```python
from build123d import *

# Parameters (mm, degrees)
SKETCH1_W           = 7
SKETCH1_H           = 7
BOSS_EXTRUDE1_DEPTH = 3
CUT_EXTRUDE1_DEPTH  = 7
CUT_EXTRUDE2_DEPTH  = 11
SKETCH4_R           = 1.8
CUT_EXTRUDE3_DEPTH  = 0.8
CUT_EXTRUDE4_DEPTH  = 0.4


with BuildPart() as part:
    # Sketch1 → Boss-Extrude1 (new body)
    with BuildSketch(Plane(origin=(0, 0, 0), x_dir=(1, 0, 0), z_dir=(0, 1, 0))):
        with Locations((3.5, 3.5)):
            Rectangle(SKETCH1_W, SKETCH1_H)
    extrude(amount=BOSS_EXTRUDE1_DEPTH)

    # Sketch2 → Cut-Extrude1 (cut)
    with BuildSketch(Plane.XY):
        Polygon((0, 0), (0.7, 3), (0, 3), align=None)
        Polygon((7, 0), (6.3, 3), (7, 3), align=None)
    extrude(amount=-CUT_EXTRUDE1_DEPTH, mode=Mode.SUBTRACT)

    # Sketch3 → Cut-Extrude2 (cut)
    with BuildSketch(Plane(origin=(0, 0, 0), x_dir=(0, 0, -1), z_dir=(1, 0, 0))):
        Polygon((0, 0), (0.7, 3), (0, 3), align=None)
        Polygon((7, 3), (6.3, 3), (7, 0), align=None)
    extrude(amount=CUT_EXTRUDE2_DEPTH, mode=Mode.SUBTRACT)

    # Sketch4 → Cut-Extrude3 (cut)
    with BuildSketch(Plane.XZ):
        with Locations(Location((3.5, -3.5, 0), (0, 0, 270))):
            Circle(SKETCH4_R)
    extrude(amount=-CUT_EXTRUDE3_DEPTH, mode=Mode.SUBTRACT)

    # Sketch5 → Cut-Extrude4 (cut)
    with BuildSketch(Plane(origin=(0, 3, 0), x_dir=(1, 0, 0), z_dir=(0, 1, 0))):
        with BuildLine():
            Line((2.118256711, 5.29301719), (2.791333634, 5.29301719))
            Line((2.791333634, 5.29301719), (2.791333634, 3.393678247))
            add(Edge.make_bspline(
                [(2.791333634, 3.393678247), (2.79159059, 3.357687368), (2.792081143, 3.288977364), (2.792418818, 3.190811929), (2.794287554, 3.102674552), (2.798340091, 3.024423212), (2.801121459, 2.956097816), (2.806286157, 2.897685825), (2.811438338, 2.849209985), (2.816447496, 2.820376155), (2.818677384, 2.807540427)],
                knots=[0, 0, 0, 0, 1.470600056, 2.807515117, 4.011048972, 5.072079398, 6.00911328, 6.804506435, 7.467811572, 8, 8, 8, 8], degree=3))
            add(Edge.make_bspline(
                [(2.818677384, 2.807540427), (2.827870656, 2.772937179), (2.845973369, 2.704799015), (2.895871105, 2.611655954), (2.961785309, 2.529556211), (3.029020227, 2.471005878), (3.08983939, 2.429568298), (3.141500286, 2.404348789), (3.196312159, 2.381359585), (3.255433761, 2.363720163), (3.318230563, 2.348285034), (3.385461086, 2.339360335), (3.456557942, 2.33251085), (3.505290309, 2.331828921), (3.530316005, 2.331478728)],
                knots=[0, 0, 0, 0, 1.376921055, 2.711331395, 4.038631339, 5.418057255, 6.132954575, 6.870556231, 7.630397752, 8.422890386, 9.247036838, 10.121396817, 11.035274583, 12, 12, 12, 12], degree=3))
            add(Edge.make_bspline(
                [(3.530316005, 2.331478728), (3.555564197, 2.331936651), (3.604721911, 2.332828219), (3.67595983, 2.338137813), (3.742423591, 2.348155186), (3.804072535, 2.361289897), (3.86123227, 2.37788997), (3.913446785, 2.398907615), (3.960633797, 2.424200444), (4.016077825, 2.462322988), (4.075735526, 2.516101492), (4.133148446, 2.589220237), (4.174238425, 2.669935378), (4.193511366, 2.743634339), (4.203417011, 2.807845981), (4.209452062, 2.864033397), (4.214971422, 2.927618056), (4.219983422, 2.9984258), (4.223410988, 3.07650978), (4.225264898, 3.162067474), (4.226723935, 3.255085239), (4.227057995, 3.319592414), (4.22723107, 3.353013183)],
                knots=[0, 0, 0, 0, 1.036876239, 2.018776863, 2.930845756, 3.794842666, 4.605604932, 5.371924355, 6.101864688, 6.799283669, 8.1310906, 9.382718023, 10.597336334, 11.822035891, 12.492591141, 13.265194674, 14.141890321, 15.11351293, 16.179860579, 17.351049011, 18.627594861, 20, 20, 20, 20], degree=3))
            Line((4.22723107, 3.353013183), (4.22723107, 5.29301719))
            Line((4.22723107, 5.29301719), (4.900307993, 5.29301719))
            Line((4.900307993, 5.29301719), (4.900307993, 3.462388183))
            add(Edge.make_bspline(
                [(4.900307993, 3.462388183), (4.900221723, 3.411906909), (4.900055958, 3.314908527), (4.897467772, 3.175352057), (4.891967054, 3.047314846), (4.887360678, 2.930577419), (4.878475168, 2.825437586), (4.86917207, 2.731829975), (4.85718756, 2.649770945), (4.840097538, 2.556498932), (4.811376645, 2.451853735), (4.765088439, 2.336259695), (4.705930722, 2.231093862), (4.634139223, 2.135952726), (4.550127521, 2.050458146), (4.452637717, 1.97494623), (4.342672295, 1.908498965), (4.241901685, 1.860652783), (4.154042624, 1.828434731), (4.082482889, 1.806630998), (4.005897563, 1.788473049), (3.924376469, 1.774063102), (3.837884577, 1.761913385), (3.746390484, 1.753799365), (3.650032611, 1.748735644), (3.584309093, 1.748345307), (3.550648537, 1.748145395)],
                knots=[0, 0, 0, 0, 1.415574045, 2.719986624, 3.913607924, 5.00929969, 5.995467356, 6.871900228, 7.64671288, 8.320227872, 9.530145585, 10.682614022, 11.803571353, 12.90325401, 14.015460715, 15.154679255, 16.351678057, 17.612271512, 18.275764165, 18.974412946, 19.708786676, 20.481351116, 21.295095879, 22.157200529, 23.056203067, 24, 24, 24, 24], degree=3))
            add(Edge.make_bspline(
                [(3.550648537, 1.748145395), (3.510214347, 1.748662249), (3.431887293, 1.749663472), (3.318189063, 1.754129843), (3.212251246, 1.763348604), (3.113741005, 1.775808622), (3.022699014, 1.791826383), (2.938894957, 1.810975517), (2.862997887, 1.835177319), (2.772598387, 1.869743344), (2.671833064, 1.922617774), (2.562145747, 1.993151834), (2.465859145, 2.072762044), (2.383819281, 2.160670513), (2.315237148, 2.253787937), (2.259491992, 2.350099358), (2.214819658, 2.447999484), (2.196153021, 2.516041987), (2.186966646, 2.549527606)],
                knots=[0, 0, 0, 0, 1.128613534, 2.186292659, 3.174878439, 4.095586888, 4.95671962, 5.754129884, 6.492676435, 7.178284149, 8.453103036, 9.659838108, 10.813193309, 11.929983019, 13.007587775, 14.033493319, 15.032227051, 16, 16, 16, 16], degree=3))
            add(Edge.make_bspline(
                [(2.186966646, 2.549527606), (2.181344262, 2.575890465), (2.169501722, 2.631419074), (2.156051883, 2.719698679), (2.143781668, 2.816909308), (2.135400951, 2.923165946), (2.127456798, 3.038131461), (2.121753178, 3.16202262), (2.119407844, 3.294811291), (2.118648152, 3.386432941), (2.118256711, 3.43364219)],
                knots=[0, 0, 0, 0, 0.728071598, 1.533551606, 2.411422299, 3.374601532, 4.412367648, 5.524718474, 6.72457895, 8, 8, 8, 8], degree=3))
            Line((2.118256711, 3.43364219), (2.118256711, 5.29301719))
        make_face()
    extrude(amount=-CUT_EXTRUDE4_DEPTH, mode=Mode.SUBTRACT)


solid = part.part
```
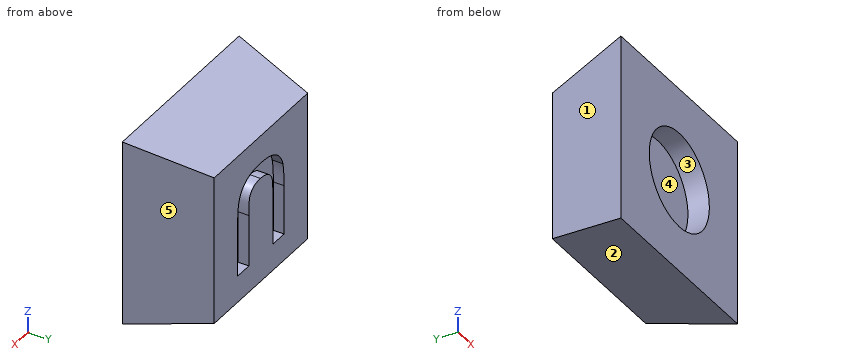
Build history of the part. All positions in model axes, mm. Face numbers are marked on the shaded views. A direction names the side the tool comes from. Give positions to 0.01 mm unless a question says otherwise; leave off trailing zeros. Order: outer loops, then holes, each group sorted by start corner. A loop starts at its lowest first (then second) coordinate and runs counter-clockwise, first axis right, second up. Notation, with made-up numbers: M 42.5,19 L 51.5,19 A13 cw 51.5,32 Z; hole C -6.5,-21 d4. An arc over 180 degrees is marked long. Return JSON: item names as keys, results as strings.
Q1. Band-saw the part on B-B (y = 0.35). Give the cut face in (x, z).
Answer list:
{"outline": "M 0.08,-6.92 L 6.92,-6.92 L 6.92,-0.08 L 0.08,-0.08 Z; hole C 3.5,-3.5 d3.6"}
Q2. Band-saw the part on C-C (x = 1.25). Give the cut face in (y, z), then the cut area to 3 significant figures.
Answer list:
{"outline": "M 0,-7 L 3,-6.3 L 3,-0.7 L 0,0 Z", "area": "18.9 mm^2"}
Q3. Two-plate mould, pull along Z, no slides. Class the marked faces 1, 2 and 3: pulls with the +Z half, pulls with the -Z half, needs draft (parallel to the pull), parting line crosses it, or undercut.
Answer list:
{"face 1": "needs draft", "face 2": "pulls with the -Z half", "face 3": "undercut"}
Q4. Wall check: probe 1 along X at (y, z) = (2.8, -2.5); probe 2 along Y at (x, z) = (3.75, -2.75); probe 3 along Z at (x, y) = (4.25, 0.65). Give the ranges that are in metal, low to high. Write a range as from..to.
Answer list:
{"probe 1": "x = 0.65..2.2, 3..4.06, 4.82..6.35", "probe 2": "y = 0.8..3", "probe 3": "z = -6.85..-5.14, -1.86..-0.15"}
Q5. Flat gauge pins, fed straight in: pin 1 (1.5 mm diameter, centred on y = 0.5, z = -3, fed in from -X); pin 2 (1.8 mm diameter, centred on x = 3.5, z = -3, fed in from -Y). Where does each tip first touch, or does it go through?
Answer list:
{"pin 1": "stops at x = 0", "pin 2": "stops at y = 0.8"}
Q6. 3-axis set-ups, long thin cutter, end or side, ignore diameter. For the marked faces 4 and 5: which of +Z, -Z, +X, -X, +Y, -Y reach the whole face in a straight line?
Answer list:
{"face 4": "-Y", "face 5": "+Z, -Z, +X, +Y"}
Q7. Band-saw the part on A-A (z = -5.5). Give the cut face in (x, y), then the cut area to 3 significant figures.
Answer list:
{"outline": "M 0,0 L 7,0 L 6.3,3 L 0.7,3 Z", "area": "18.9 mm^2"}
